Source: CAD feature listing. Evaluate the final solid. Frame: model axes, mm. Round coordinates to 2 decimals unless told otherwise and drop trailing zeros. Order: outer loops, then holes, each group sorted by start corner. A loop starts at its lowest first (then second) coordinate and runs counter-clockwise, first axis right, second up. Notation, with made-up numbers: (64, 74) -> (102, 74) arc R29 ccw to (102, 106) -> close; hole circle Ø5 at (80, 76.25). An arc over 180 degrees is marked (long way). Write item = value, one per line. Start each with the question number.
(1) Draft query along X for faces 1 (the face through (-136.505, -78.566, 7.465)), 2 (the face through (-71.7, -124.7, 7.5)), 3 (the face through (-153.89, -28.73, 7.46)), 4 (the face through (-137, -79, 5)). Return one class per face: released by +X, released by -X, zero draft, split by the parting line, or undercut.
(2) Contact query for flat-ended pins moving along their axis: pin 1 Ø1.5 at (x, z) = (-44.5, 6.5) entering from +Y; pin 2 Ø1 at (x, z) = (-103.5, 8) entering from -Y; pin 3 Ø1.5 at (y, z) = (-76.5, 7) entering from -X. Output: stop coordinate, or through.
(3) Ray query, line 1 (X direction, y = -5.5, z = 9.7); line 2 (Y direction, x = -42.5, z = 9.5); line 3 (X direction, y = -59.5, z = 6.8). Return the intervals inside material, ascending.
(4) Cut plane C-C on y = -48.5. Return the cut outline in (x, z), then the cut area to 3 significant figures.
(5) Cut plane A-A on z = 8.6. Return the cut outline in (x, y).
(6) Cut plane B-B on x = -61. Return the cut outline in (y, z), then the cut area to 3 significant figures.
Solid Edge part; units mm, degrees
sketch "Sketch1" plane through (0.0007, 14.651, 5) normal (0, 0, 1) x (1, 0, 0)
  line L0 (-114.0407, 98.8093) -> (-57.2599, 131.5929)
  arc A0 (-54.1474, 131.5247) -> (-57.2599, 131.5929) centre (-55.7598, 128.9948) ccw
  arc A1 (-47.0142, 137.1861) -> (-48.7662, 134.4664) centre (-45.7662, 134.458) ccw
  arc A2 (-47.0142, 137.1861) -> (-26.9146, 142.5706) centre (-21.0226, 80.3698) cw
  arc A3 (-24.0376, 141.0909) -> (-26.9146, 142.5706) centre (-26.6317, 139.5839) ccw
  arc A4 (-15.245, 142.849) -> (-17.9063, 141.2336) centre (-15.245, 139.849) ccw
  line L1 (-15.245, 142.849) -> (15.2436, 142.849)
  arc A5 (17.905, 141.2336) -> (15.2436, 142.849) centre (15.2436, 139.849) ccw
  arc A6 (26.9132, 142.5696) -> (24.036, 141.0904) centre (26.6298, 139.583) ccw
  arc A7 (26.9132, 142.5696) -> (47.0027, 137.1869) centre (21.0099, 80.3561) cw
  arc A8 (48.7549, 134.4673) -> (47.0027, 137.1869) centre (45.7549, 134.4587) ccw
  arc A9 (57.2487, 131.5943) -> (54.1362, 131.526) centre (55.7487, 128.9962) ccw
  line L2 (57.2487, 131.5943) -> (114.0299, 98.8129)
  arc A10 (115.5271, 96.0833) -> (114.0299, 98.8129) centre (112.5299, 96.2148) ccw
  arc A11 (124.0003, 92.7805) -> (120.7849, 92.9052) centre (122.2944, 90.3127) ccw
  arc A12 (124.0003, 92.7805) -> (155.0355, 39.027) centre (82.7747, 33.1424) cw
  arc A13 (153.5358, 36.1799) -> (155.0355, 39.027) centre (152.0454, 38.7835) ccw
  arc A14 (155.2747, 27.3761) -> (153.6593, 30.0375) centre (152.2747, 27.3761) ccw
  line L3 (155.2747, 27.3761) -> (155.2747, -38.192)
  arc A15 (153.6593, -40.8534) -> (155.2747, -38.192) centre (152.2747, -38.192) ccw
  arc A16 (154.9954, -49.8615) -> (153.5161, -46.9844) centre (152.0088, -49.5782) ccw
  arc A17 (154.9954, -49.8615) -> (149.6134, -69.9554) centre (92.7533, -43.9583) cw
  arc A18 (146.8942, -71.7079) -> (149.6134, -69.9554) centre (146.8851, -68.7079) ccw
  arc A19 (144.0217, -80.2016) -> (143.9534, -77.0892) centre (141.4236, -78.7016) ccw
  line L4 (144.0217, -80.2016) -> (127.6444, -108.5679)
  arc A20 (122.7007, -116.5716) -> (122.8583, -113.3403) centre (120.256, -114.8329) ccw
  arc A21 (77.6703, -142.5696) -> (122.7007, -116.5716) centre (71.767, -80.3476) ccw
  arc A22 (74.7931, -141.0904) -> (77.6703, -142.5696) centre (77.3869, -139.583) ccw
  arc A23 (66.0007, -142.849) -> (68.6621, -141.2336) centre (66.0007, -139.849) ccw
  line L5 (5.7656, -142.849) -> (66.0007, -142.849)
  arc A24 (3.1042, -141.2336) -> (5.7656, -142.849) centre (5.7656, -139.849) ccw
  arc A25 (-5.767, -142.849) -> (-3.1056, -141.2336) centre (-5.767, -139.849) ccw
  line L6 (-66.0021, -142.849) -> (-5.767, -142.849)
  arc A26 (-68.6634, -141.2336) -> (-66.0021, -142.849) centre (-66.0021, -139.849) ccw
  arc A27 (-77.6716, -142.5694) -> (-74.7944, -141.0903) centre (-77.3881, -139.5828) ccw
  arc A28 (-122.6994, -116.5717) -> (-77.6716, -142.5694) centre (-71.7665, -80.349) ccw
  arc A29 (-122.857, -113.3404) -> (-122.6994, -116.5717) centre (-120.2547, -114.833) ccw
  arc A30 (-128.7762, -106.6053) -> (-126.0465, -108.1024) centre (-126.1781, -105.1053) ccw
  line L7 (-144.0218, -80.199) -> (-128.7762, -106.6053)
  arc A31 (-143.9535, -77.0865) -> (-144.0218, -80.199) centre (-141.4237, -78.699) ccw
  arc A32 (-149.6144, -69.9531) -> (-146.8949, -71.7053) centre (-146.8862, -68.7053) ccw
  arc A33 (-154.9987, -49.8585) -> (-149.6144, -69.9531) centre (-92.7672, -43.9523) ccw
  arc A34 (-153.5196, -46.9813) -> (-154.9987, -49.8585) centre (-152.0122, -49.5751) ccw
  arc A35 (-155.2786, -38.189) -> (-153.6631, -40.8503) centre (-152.2786, -38.1889) ccw
  line L8 (-155.2818, 27.3758) -> (-155.2786, -38.189)
  arc A36 (-153.6665, 30.0373) -> (-155.2818, 27.3758) centre (-152.2818, 27.376) ccw
  arc A37 (-155.0428, 39.0267) -> (-153.5432, 36.1796) centre (-152.0527, 38.7832) ccw
  arc A38 (-124.0109, 92.7765) -> (-155.0428, 39.0267) centre (-82.7847, 33.1421) ccw
  arc A39 (-120.7955, 92.9014) -> (-124.0109, 92.7765) centre (-122.3049, 90.3088) ccw
  arc A40 (-114.0407, 98.8093) -> (-115.5378, 96.0796) centre (-112.5406, 96.2112) ccw
  arc A41 (-48.7662, 134.4664) -> (-54.1474, 131.5247) centre (-52.2662, 134.4761) cw
  arc A42 (-17.9064, 141.2336) -> (-24.0377, 141.0909) centre (-21.0113, 142.849) cw
  arc A43 (24.036, 141.0904) -> (17.905, 141.2336) centre (21.0099, 142.849) cw
  arc A44 (54.1362, 131.526) -> (48.7549, 134.4673) centre (52.2549, 134.4774) cw
  arc A45 (120.7849, 92.9052) -> (115.5271, 96.0832) centre (119.0237, 95.9298) cw
  arc A46 (153.6593, 30.0375) -> (153.5358, 36.1799) centre (155.2747, 33.1424) cw
  arc A47 (153.5161, -46.9844) -> (153.6593, -40.8534) centre (155.2747, -43.9583) cw
  arc A48 (143.9534, -77.0891) -> (146.8942, -71.7079) centre (146.9048, -75.2079) cw
  arc A49 (122.8584, -113.3404) -> (127.6444, -108.5679) centre (125.8944, -111.599) cw
  arc A50 (68.6621, -141.2336) -> (74.7931, -141.0904) centre (71.767, -142.849) cw
  arc A51 (-3.1056, -141.2336) -> (3.1042, -141.2336) centre (-0.0007, -142.849) cw
  arc A52 (-74.7944, -141.0903) -> (-68.6635, -141.2336) centre (-71.7684, -142.849) cw
  arc A53 (-126.0466, -108.1024) -> (-122.857, -113.3404) centre (-125.8931, -111.599) cw
  arc A54 (-146.8949, -71.7053) -> (-143.9536, -77.0866) centre (-146.905, -75.2053) cw
  arc A55 (-153.6632, -40.8503) -> (-153.5196, -46.9813) centre (-155.2784, -43.9553) cw
  arc A56 (-153.5432, 36.1796) -> (-153.6665, 30.0373) centre (-155.2821, 33.1421) cw
  arc A57 (-115.5377, 96.0796) -> (-120.7955, 92.9014) centre (-119.0344, 95.926) cw
  line L9 (-56.0166, 140.971) -> (-122.7845, 102.4212)
  arc A58 (-162.7821, 33.1421) -> (-122.7845, 102.4212) centre (-82.7847, 33.1421) cw
  line L10 (-162.7821, 33.1421) -> (-162.7784, -43.9553)
  arc A59 (-162.7784, -43.9553) -> (-153.4002, -78.9553) centre (-92.7784, -43.9553) ccw
  line L11 (-132.3882, -115.349) -> (-153.4002, -78.9553)
  arc A60 (-132.3882, -115.349) -> (-71.7683, -150.349) centre (-71.7665, -80.349) ccw
  line L12 (71.767, -150.349) -> (-71.7683, -150.349)
  arc A61 (71.767, -150.349) -> (132.3896, -115.349) centre (71.7678, -80.349) ccw
  line L13 (132.3896, -115.349) -> (153.4002, -78.9576)
  arc A62 (162.7747, -43.9583) -> (153.4002, -78.9576) centre (92.791, -43.9684) cw
  line L14 (162.7747, 33.1424) -> (162.7747, -43.9583)
  arc A63 (122.7736, 102.4251) -> (162.7747, 33.1424) centre (82.7747, 33.1424) cw
  line L15 (56.0045, 140.9728) -> (122.7736, 102.4251)
  arc A64 (21.0099, 150.349) -> (56.0045, 140.9728) centre (21.008, 80.349) cw
  line L16 (-21.0112, 150.349) -> (21.0099, 150.349)
  arc A65 (-32.5074, 149.4015) -> (-21.0112, 150.349) centre (-20.997, 79.961) cw
  arc A66 (-44.641, 146.2432) -> (-32.5074, 149.4015) centre (-21.0122, 80.3518) cw
  arc A67 (-56.0166, 140.971) -> (-44.641, 146.2432) centre (-21.0122, 80.3518) cw
  circle A68 centre (-71.7683, -142.849) radius 1.5
  circle A69 centre (-0.0007, -142.849) radius 1.5
  circle A70 centre (-125.893, -111.599) radius 1.5
  circle A71 centre (-146.905, -75.2053) radius 1.5
  circle A72 centre (-155.2784, -43.9553) radius 1.5
  circle A73 centre (-155.2821, 33.1421) radius 1.5
  circle A74 centre (-119.0344, 95.9261) radius 1.5
  circle A75 centre (-52.2662, 134.4761) radius 1.5
  circle A76 centre (-21.0112, 142.849) radius 1.5
  circle A77 centre (21.0099, 142.849) radius 1.5
  circle A78 centre (52.2549, 134.4774) radius 1.5
  circle A79 centre (119.0237, 95.9298) radius 1.5
  circle A80 centre (155.2747, 33.1424) radius 1.5
  circle A81 centre (155.2747, -43.9583) radius 1.5
  circle A82 centre (146.9048, -75.2079) radius 1.5
  circle A83 centre (125.8944, -111.599) radius 1.5
  circle A84 centre (71.767, -142.849) radius 1.5
extrude "ExtrudedProtrusion_7" add sketch "Sketch1" along normal blind 5
sketch "Sketch2" plane through (-0.003, 14.651, 10) normal (0, 0, 1) x (1, 0, 0)
  line L0 (-168.1883, -5.4066) -> (170.0115, -5.4066)
  line L1 (170.0115, -5.4066) -> (170.0115, 153.6029)
  line L2 (170.0115, 153.6029) -> (-168.1883, 153.6029)
  line L3 (-168.1883, 153.6029) -> (-168.1883, -5.4066)
extrude "Cutout1" cut sketch "Sketch2" against normal up to next
sketch "Sketch3" plane through (-0.0021, -63.2268, 10) normal (0, 0, 1) x (1, 0, 0)
  line L0 (-35.8817, -72.4712) -> (180.5414, -72.4712)
  line L1 (180.5414, -72.4712) -> (180.5414, 89.6223)
  line L2 (180.5414, 89.6223) -> (-35.8817, 89.6223)
  line L3 (-35.8817, 89.6223) -> (-35.8817, -72.4712)
extrude "Cutout2" cut sketch "Sketch3" against normal up to next
properties material "Polycarbonate"
Evaluation:
q1.face_1 = released by +X
q1.face_2 = undercut
q1.face_3 = undercut
q1.face_4 = zero draft
q2.pin_1 = -128.2
q2.pin_2 = -128.34
q2.pin_3 = -146.79
q3.line_1 = -162.78 to -155.28
q3.line_2 = -135.7 to -128.2
q3.line_3 = -155.93 to -147.97, -145.84 to -143.57
q4.outline = (-160.09, 5) -> (-152.26, 5) -> (-152.26, 10) -> (-160.09, 10) -> close
q4.area = 39.2 mm^2
q5.outline = (-162.78, -29.3) arc R70 ccw to (-153.4, -64.3) -> (-132.39, -100.7) arc R70 ccw to (-71.77, -135.7) -> (-35.88, -135.7) -> (-35.88, -128.2) -> (-66, -128.2) arc R3 cw to (-68.66, -126.58) arc R3.5 ccw to (-74.79, -126.44) arc R3 cw to (-77.67, -127.92) arc R62.5 cw to (-122.7, -101.92) arc R3 cw to (-122.86, -98.69) arc R3.5 ccw to (-126.05, -93.45) arc R3 cw to (-128.78, -91.95) -> (-144.02, -65.55) arc R3 cw to (-143.95, -62.44) arc R3.5 ccw to (-146.89, -57.05) arc R3 cw to (-149.61, -55.3) arc R62.51 cw to (-155, -35.21) arc R3 cw to (-153.52, -32.33) arc R3.5 ccw to (-153.66, -26.2) arc R3 cw to (-155.28, -23.54) -> (-155.28, 9.24) -> (-162.78, 9.24) -> close; hole circle Ø3 at (-155.28, -29.3); hole circle Ø3 at (-146.9, -60.55); hole circle Ø3 at (-125.89, -96.95); hole circle Ø3 at (-71.77, -128.2)
q6.outline = (-135.7, 5) -> (-128.2, 5) -> (-128.2, 10) -> (-135.7, 10) -> close
q6.area = 37.5 mm^2
